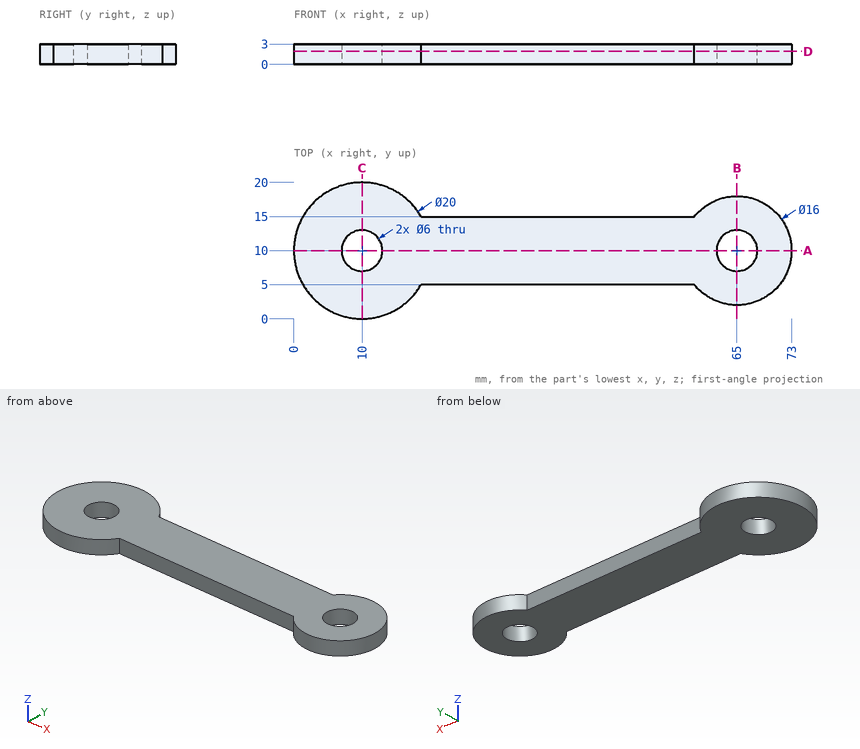
Drawing for the job (mm, zero at the part's lowest x, y, z). Round coordinates to 2 decimals unless told otherwise and drop trailing zeros. Write each loop counter-clockwise with the first axis right and the second up, starting at its lowest first coordinate (ties: lowest second). Pieces come first, ordered by that corner, then holes. Notation, with made-up numbers: (-5.5, 89) - (14.5, 89) arc R24 ccw to (14.5, 128) - close; hole circle Ø8 at (-39, 12). An arc over 180 degrees is marked (long way). Return JSON: item names as keys, results as strings. Group by question number.
Item 1: Band-saw the part on B-B on x = 65. List the corners of the cut face in (y, z), plus the area to 3 significant figures.
Item 2: Flat gauge pins, fed straight in: pin 1 Ø0.9 at (x, z) = (46.5, 1) entering from +Y; pin 2 Ø3 at (x, y) = (18.5, 18) entering from +Z; pin 3 Ø1.5 at (x, z) = (45.5, 1) entering from -Y. Where does each tip first touch, or does it go through?
Item 3: Band-saw the part on A-A on y = 10. List the corners of the cut face in (x, z), plus the area to 3 significant figures.
Item 4: Band-saw the part on C-C on x = 10. List the corners of the cut face in (y, z).
Item 5: Band-saw the part on D-D on z = 1.9. List the corners of the cut face in (x, y) (3 decimals).
Item 6: Probe probe 1 along X at (y, z) = (7.5, 1.85); probe 2 along Y at (x, z) = (10, 1.65); probe 3 along X at (y, z) = (8, 1.5). List the from-to ranges inside material, lowest first.
Resolved:
{
 "1": {"outline": "(2, 0) - (7, 0) - (7, 3) - (2, 3) - close; (13, 0) - (18, 0) - (18, 3) - (13, 3) - close", "area": "30.0 mm²"},
 "2": {"pin 1": "stops at y = 15", "pin 2": "passes through", "pin 3": "stops at y = 5"},
 "3": {"outline": "(0, 0) - (7, 0) - (7, 3) - (0, 3) - close; (13, 0) - (62, 0) - (62, 3) - (13, 3) - close; (68, 0) - (73, 0) - (73, 3) - (68, 3) - close", "area": "183 mm²"},
 "4": {"outline": "(0, 0) - (7, 0) - (7, 3) - (0, 3) - close; (13, 0) - (20, 0) - (20, 3) - (13, 3) - close"},
 "5": {"outline": "(18.66, 5) - (58.755, 5) arc R8 ccw (long way) to (58.755, 15) - (18.66, 15) arc R10 ccw (long way) to start; hole circle Ø6 at (10, 10); hole circle Ø6 at (65, 10)"},
 "6": {"probe 1": "x = 0.32 to 8.34, 11.66 to 63.34, 66.66 to 72.6", "probe 2": "y = 0 to 7, 13 to 20", "probe 3": "x = 0.2 to 7.76, 12.24 to 62.76, 67.24 to 72.75"}
}
